Geometry: see drawing. Coordinates: mm, zero at the bounding-box minimum. A direction names the side the tool comes from. Coordinates: 2 decimals unless noted, no trailing zeros. Order: outer loops, then holes, each group sorted by start corner. A loop starts at its lowest first (then second) coordinate and runs counter-clockwise, first axis right, second up.
Item 1: Reachability of the marked faces 4, 5 and 6 from +Z, -Z, +X, -X, +Y, -Y: full face, straight path, thin tool, end or side. Return the list, or none.
Item 2: Section B-B on y = 5.08. State how many separate pieces and enclosed holes the cut face has, then the cut area to 3 significant figures.
Item 3: Section A-A on y = 35.5. Return the cut outline in (x, z) (3 decimals), then the cut area to 3 significant figures.
Item 4: Ray query, line 1 (Z direction, x = 53, y = 37); line 2 (Y direction, x = 34.75, z = 82.55) (3 decimals); line 3 (Z direction, x = 21, y = 5). Return the intervals inside material, ascending.
Item 5: Contact query for flat-ended pins moving along their axis: P1, Ø4, axis at y = 6.35, z = 9.525, coming from the +X side; P2, Ø16, axis at y = 15, z = 39.5, coming from the -X side; P3, Ø14.5, axis at y = 22.225, z = 82.55, coming from the -X side; P4, Ø4, axis at y = 5.5, z = 61, coming from the +X side. Output: stop coordinate, or through.
Item 6: Section D-D on z = 62. Return the cut outline in (x, y).
Item 7: Section C-C on z = 82.55. Return the cut outline in (x, y) (3 decimals).
Item 8: Mould query, pull axis Z, two halves, no side actions, for the marked faces 1, 2 and 3. Classes: released by +Z, released by -Z, zero draft, split by the parting line, or undercut.
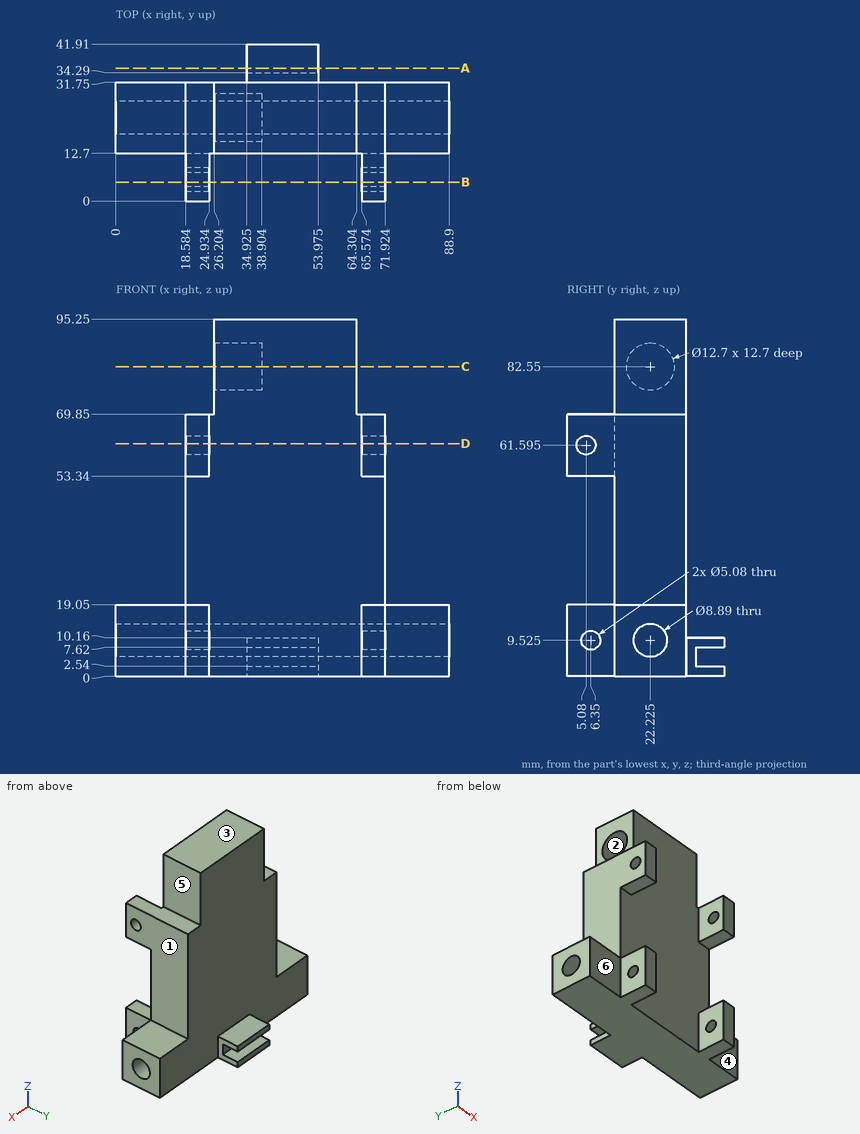
Answer list:
1. face 4: +Z, -Z, +X, -Y
1. face 5: +Z, +X, +Y, -Y
1. face 6: +Z, -Z, -X, -Y
2. separate pieces: 8
2. enclosed holes: 0
2. area: 331 mm2
3. outline: (34.925, 0) - (53.975, 0) - (53.975, 2.54) - (34.925, 2.54) - close; (34.925, 7.62) - (53.975, 7.62) - (53.975, 10.16) - (34.925, 10.16) - close
3. area: 96.8 mm2
4. line 1: z = 0 to 2.54, 7.62 to 10.16
4. line 2: y = 12.7 to 15.875, 28.575 to 31.75
4. line 3: z = 0 to 7.37, 11.68 to 19.05, 53.34 to 59.06, 64.13 to 69.85
5. P1: passes through
5. P2: stops at x = 18.58
5. P3: stops at x = 26.2
5. P4: stops at x = 71.92
6. outline: (18.58, 0) - (24.93, 0) - (24.93, 2.57) - (18.58, 2.57) - close; (18.58, 7.59) - (24.93, 7.59) - (24.93, 12.7) - (65.57, 12.7) - (65.57, 7.59) - (71.92, 7.59) - (71.92, 31.75) - (18.58, 31.75) - close; (65.57, 0) - (71.92, 0) - (71.92, 2.57) - (65.57, 2.57) - close
7. outline: (26.204, 12.7) - (64.304, 12.7) - (64.304, 31.75) - (26.204, 31.75) - (26.204, 28.575) - (38.904, 28.575) - (38.904, 15.875) - (26.204, 15.875) - close
8. face 1: zero draft
8. face 2: undercut
8. face 3: released by +Z
